```python
from build123d import *

# Parameters (mm, degrees)
SKETCH_1_W      = 60
SKETCH_1_H      = 42
SKETCH_1_R      = 1.05
SKETCH_1_R_2    = 1.55
SKETCH_1_W_2    = 20
SKETCH_1_H_2    = 15
EXTRUDE_1_DEPTH = 3


with BuildPart() as part:
    # 草图1 → 凸台-拉伸1 (new body)
    with BuildSketch(Plane.XY):
        Rectangle(SKETCH_1_W, SKETCH_1_H)
        with Locations((-18, -8.5)):
            Circle(SKETCH_1_R, mode=Mode.SUBTRACT)
        with Locations((-18, 8.5)):
            Circle(SKETCH_1_R, mode=Mode.SUBTRACT)
        with Locations((18, 8.5)):
            Circle(SKETCH_1_R, mode=Mode.SUBTRACT)
        with Locations((18, -8.5)):
            Circle(SKETCH_1_R, mode=Mode.SUBTRACT)
        with Locations((-27, -18)):
            Circle(SKETCH_1_R_2, mode=Mode.SUBTRACT)
        with Locations((27, -18)):
            Circle(SKETCH_1_R_2, mode=Mode.SUBTRACT)
        with Locations((27, 18)):
            Circle(SKETCH_1_R_2, mode=Mode.SUBTRACT)
        with Locations((-27, 18)):
            Circle(SKETCH_1_R_2, mode=Mode.SUBTRACT)
        Rectangle(SKETCH_1_W_2, SKETCH_1_H_2, mode=Mode.SUBTRACT)
        with BuildLine():
            Line((-10, 17.5), (10, 17.5))
            ThreePointArc((10, 17.5), (12.5, 15), (10, 12.5))
            Line((10, 12.5), (-10, 12.5))
            ThreePointArc((-10, 12.5), (-12.5, 15), (-10, 17.5))
        make_face(mode=Mode.SUBTRACT)
        with BuildLine():
            Line((-10, -17.5), (10, -17.5))
            ThreePointArc((10, -17.5), (12.5, -15), (10, -12.5))
            Line((10, -12.5), (-10, -12.5))
            ThreePointArc((-10, -12.5), (-12.5, -15), (-10, -17.5))
        make_face(mode=Mode.SUBTRACT)
        with BuildLine():
            Line((-23.583325542, 10), (-23.583325542, -10))
            ThreePointArc((-23.583325542, -10), (-25.133325542, -11.55), (-26.683325542, -10))
            Line((-26.683325542, -10), (-26.683325542, 10))
            ThreePointArc((-26.683325542, 10), (-25.133325542, 11.55), (-23.583325542, 10))
        make_face(mode=Mode.SUBTRACT)
        with BuildLine():
            Line((23.583325542, 10), (23.583325542, -10))
            ThreePointArc((23.583325542, -10), (25.133325542, -11.55), (26.683325542, -10))
            Line((26.683325542, -10), (26.683325542, 10))
            ThreePointArc((26.683325542, 10), (25.133325542, 11.55), (23.583325542, 10))
        make_face(mode=Mode.SUBTRACT)
    extrude(amount=EXTRUDE_1_DEPTH)


solid = part.part
```
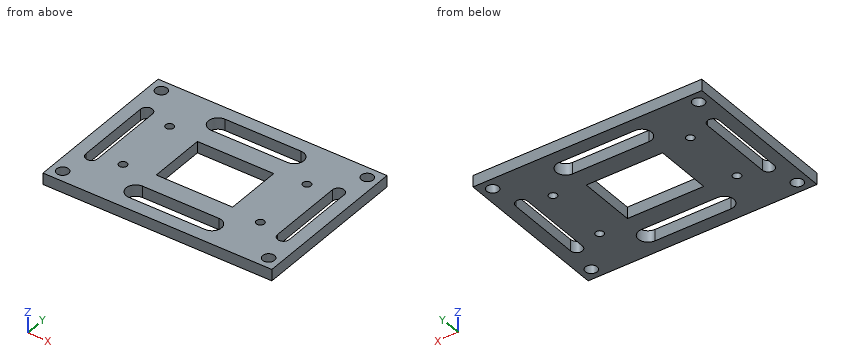
The listing builds one solid part. Answer for the finished solid, in the listing's coordinates (mm). Round coordinates to 2 decimals unless told otherwise and drop trailing zeros. Loops run counter-clockwise (first coordinate to the right, second up) from the corner with the lowest first, then second, coordinate; pieces in that order, holes last. Notation, with made-up numbers: (-13.5, 51.25) - (-1.5, 51.25) arc R10 cw to (-1.5, 69.25) - close; hole circle Ø3 at (53.25, 30.25). An arc over 180 degrees is marked (long way). Return JSON: item names as keys, results as strings. Group by question number.
1. The part is cut by section B-B on z = 1.5. State how many separate pieces and enclosed holes the cut face has, then the cut area to 3 significant figures.
2. The part is cut by section C-C on y = 15. Determine the outline of the cut face in (x, z), then the cut area to 3 significant figures.
3. Consider probe 1 along X at (y, z) = (1, 1.8); probe 2 along Y at (x, z) = (-18, 1.3); probe 3 along Y at (x, z) = (2.5, 1.15). Determine where each line is inside the solid, lowest interval first.
4. The part is cut by section A-A on y = -2. Determine the outline of the cut face in (x, z).
Resolved:
{
 "1": {"separate pieces": "1", "enclosed holes": "13", "area": "1,800 mm²"},
 "2": {"outline": "(-30, 0) - (-12.5, 0) - (-12.5, 3) - (-30, 3) - close; (12.5, 0) - (30, 0) - (30, 3) - (12.5, 3) - close", "area": "105 mm²"},
 "3": {"probe 1": "x = -30 to -26.68, -23.58 to -10, 10 to 23.58, 26.68 to 30", "probe 2": "y = -21 to -9.55, -7.45 to 7.45, 9.55 to 21", "probe 3": "y = -21 to -17.5, -12.5 to -7.5, 7.5 to 12.5, 17.5 to 21"},
 "4": {"outline": "(-30, 0) - (-26.68, 0) - (-26.68, 3) - (-30, 3) - close; (-23.58, 0) - (-10, 0) - (-10, 3) - (-23.58, 3) - close; (10, 0) - (23.58, 0) - (23.58, 3) - (10, 3) - close; (26.68, 0) - (30, 0) - (30, 3) - (26.68, 3) - close"}
}
